from build123d import *

# Parameters (mm, degrees)
SKETCH1_W               = 80
SKETCH1_H               = 90
BOSS_EXTRUDE1_DEPTH     = 6
SKETCH4_W               = 80
SKETCH4_H               = 90
SKETCH4_W_2             = 73
SKETCH4_H_2             = 83
BOSS_EXTRUDE2_DEPTH     = 54
SKETCH6_R               = 4.05
SKETCH6_R_2             = 5
CUT_EXTRUDE1_DEPTH      = 40
SKETCH7_R               = 7
CUT_EXTRUDE2_DEPTH      = 2.8
BOSS_EXTRUDE3_DEPTH     = 7
SKETCH11_R              = 2.85
BOSS_EXTRUDE4_DEPTH     = 2
CUT_EXTRUDE3_DEPTH      = 9
CUT_EXTRUDE3_DEPTH_BACK = 6
SKETCH5_R               = 1.5
CUT_EXTRUDE4_DEPTH      = 6
CUT_EXTRUDE4_DEPTH_BACK = 81.876448982
SKETCH12_W              = 33
SKETCH12_H              = 13.5
CUT_EXTRUDE6_DEPTH      = 3.5
SKETCH17_R              = 8
CUT_EXTRUDE8_DEPTH      = 2
CUT_EXTRUDE9_DEPTH      = 1.5
CUT_EXTRUDE10_DEPTH     = 10
BOSS_EXTRUDE5_DEPTH     = 90
BOSS_EXTRUDE5_2_DEPTH   = 90
SKETCH21_W              = 3.5
SKETCH21_H              = 8
BOSS_EXTRUDE6_DEPTH     = 80
SKETCH22_W              = 80
SKETCH22_H              = 3.5
BOSS_EXTRUDE7_DEPTH     = 4.5
SKETCH24_W              = 8
SKETCH24_H              = 3.5
BOSS_EXTRUDE8_DEPTH     = 90


with BuildPart() as part:
    # Sketch1 → Boss-Extrude1 (new body)
    with BuildSketch(Plane(origin=(0, 0, 0), x_dir=(1, 0, 0), z_dir=(0, 1, 0))):
        Rectangle(SKETCH1_W, SKETCH1_H)
    extrude(amount=BOSS_EXTRUDE1_DEPTH)

    # Sketch4 → Boss-Extrude2 (add)
    with BuildSketch(Plane(origin=(0, 6, 0), x_dir=(1, 0, 0), z_dir=(0, 1, 0))):
        Rectangle(SKETCH4_W, SKETCH4_H)
        Rectangle(SKETCH4_W_2, SKETCH4_H_2, mode=Mode.SUBTRACT)
    extrude(amount=BOSS_EXTRUDE2_DEPTH)

    # Sketch6 → Cut-Extrude1 (cut)
    with BuildSketch(Plane(origin=(0, 6, 0), x_dir=(1, 0, 0), z_dir=(0, 1, 0))):
        with Locations(Location((-20, 25, 0), (0, 0, 270))):
            Circle(SKETCH6_R)
        with Locations(Location((-20, -25, 0), (0, 0, 270))):
            Circle(SKETCH6_R)
        with Locations(Location((20, -25, 0), (0, 0, 270))):
            Circle(SKETCH6_R_2)
    extrude(amount=-CUT_EXTRUDE1_DEPTH, mode=Mode.SUBTRACT)

    # Sketch7 → Cut-Extrude2 (cut)
    with BuildSketch(Plane(origin=(0, 6, 0), x_dir=(1, 0, 0), z_dir=(0, 1, 0))):
        with Locations(Location((-20, 25, 0), (0, 0, 270))):
            Circle(SKETCH7_R)
        with Locations(Location((-20, -25, 0), (0, 0, 270))):
            Circle(SKETCH7_R)
    extrude(amount=-CUT_EXTRUDE2_DEPTH, mode=Mode.SUBTRACT)

    # Sketch10 → Boss-Extrude3 (add)
    with BuildSketch(Plane(origin=(0, 6, 0), x_dir=(1, 0, 0), z_dir=(0, 1, 0))):
        Polygon((-32.5, 29.600297611), (-37.35, 26.800148806), (-37.35, 21.199851194), (-32.5, 18.399702389), (-27.65, 21.199851194), (-27.65, 26.800148806), align=None)
        Polygon((2.8, 19.600297611), (-2.05, 16.800148806), (-2.05, 11.199851194), (2.8, 8.399702389), (7.65, 11.199851194), (7.65, 16.800148806), align=None)
        Polygon((2.8, -8.399702389), (-2.05, -11.199851194), (-2.05, -16.800148806), (2.8, -19.600297611), (7.65, -16.800148806), (7.65, -11.199851194), align=None)
        Polygon((-27.65, -21.199851194), (-32.5, -18.399702389), (-37.35, -21.199851194), (-37.35, -26.800148806), (-32.5, -29.600297611), (-27.65, -26.800148806), align=None)
    extrude(amount=BOSS_EXTRUDE3_DEPTH)

    # Sketch11 → Boss-Extrude4 (add)
    with BuildSketch(Plane(origin=(0, 13, 0), x_dir=(1, 0, 0), z_dir=(0, 1, 0))):
        with Locations(Location((-32.5, 24, 0), (0, 0, 270))):
            Circle(SKETCH11_R)
        with Locations(Location((2.8, 14, 0), (0, 0, 270))):
            Circle(SKETCH11_R)
        with Locations(Location((2.8, -14, 0), (0, 0, 270))):
            Circle(SKETCH11_R)
        with Locations(Location((-32.5, -24, 0), (0, 0, 270))):
            Circle(SKETCH11_R)
    extrude(amount=BOSS_EXTRUDE4_DEPTH)

    # Sketch5 → Cut-Extrude3 (cut, two sides: drawn at the far end of the back side and taken through both)
    with BuildSketch(Plane(origin=(0, 6, 0), x_dir=(1, 0, 0), z_dir=(0, 1, 0)).offset(-CUT_EXTRUDE3_DEPTH_BACK)):
        with Locations(Location((-32.5, 24, 0), (0, 0, 270))):
            Circle(SKETCH5_R)
        with Locations(Location((-32.5, -24, 0), (0, 0, 270))):
            Circle(SKETCH5_R)
        with Locations(Location((2.8, 14, 0), (0, 0, 270))):
            Circle(SKETCH5_R)
        with Locations(Location((2.8, -14, 0), (0, 0, 270))):
            Circle(SKETCH5_R)
    extrude(amount=CUT_EXTRUDE3_DEPTH + CUT_EXTRUDE3_DEPTH_BACK, mode=Mode.SUBTRACT)

    # Sketch8 → Cut-Extrude4 (cut, two sides: drawn at the far end of the back side and taken through both)
    with BuildSketch(Plane(origin=(0, 6, 0), x_dir=(1, 0, 0), z_dir=(0, 1, 0)).offset(-CUT_EXTRUDE4_DEPTH_BACK)):
        Polygon((-29.65, 25.645448267), (-32.5, 27.290896534), (-35.35, 25.645448267), (-35.35, 22.354551733), (-32.5, 20.709103466), (-29.65, 22.354551733), align=None)
        Polygon((-29.65, -22.354551733), (-32.5, -20.709103466), (-35.35, -22.354551733), (-35.35, -25.645448267), (-32.5, -27.290896534), (-29.65, -25.645448267), align=None)
        Polygon((5.65, -12.354551733), (2.8, -10.709103466), (-0.05, -12.354551733), (-0.05, -15.645448267), (2.8, -17.290896534), (5.65, -15.645448267), align=None)
        Polygon((5.65, 15.645448267), (2.8, 17.290896534), (-0.05, 15.645448267), (-0.05, 12.354551733), (2.8, 10.709103466), (5.65, 12.354551733), align=None)
    extrude(amount=CUT_EXTRUDE4_DEPTH + CUT_EXTRUDE4_DEPTH_BACK, mode=Mode.SUBTRACT)

    # Sketch12 → Cut-Extrude6 (cut)
    with BuildSketch(Plane(origin=(-36.5, 0, 0), x_dir=(0, 0, -1), z_dir=(1, 0, 0))):
        with Locations((0, 23.25)):
            Rectangle(SKETCH12_W, SKETCH12_H)
    extrude(amount=-CUT_EXTRUDE6_DEPTH, mode=Mode.SUBTRACT)

    # Sketch17 → Cut-Extrude8 (cut)
    with BuildSketch(Plane.ZY.offset(40)):
        with Locations((0, 45.25)):
            Circle(SKETCH17_R)
    extrude(amount=-CUT_EXTRUDE8_DEPTH, mode=Mode.SUBTRACT)

    # Sketch15 → Cut-Extrude9 (cut)
    with BuildSketch(Plane(origin=(-36.5, 0, 0), x_dir=(0, 0, -1), z_dir=(1, 0, 0))):
        Polygon((-6.495190528, 56.5), (-12.990381057, 45.25), (-6.495190528, 34), (6.495190528, 34), (12.990381057, 45.25), (6.495190528, 56.5), align=None)
    extrude(amount=-CUT_EXTRUDE9_DEPTH, mode=Mode.SUBTRACT)

    # Sketch19 → Cut-Extrude10 (cut)
    with BuildSketch(Plane(origin=(0, 6, 0), x_dir=(1, 0, 0), z_dir=(0, 1, 0))):
        with BuildLine():
            Line((-3.5, -5.5), (-3.5, 5.5))
            ThreePointArc((-3.5, 5.5), (0, 9), (3.5, 5.5))
            Line((3.5, 5.5), (3.5, -5.5))
            ThreePointArc((3.5, -5.5), (0, -9), (-3.5, -5.5))
        make_face()
    extrude(amount=-CUT_EXTRUDE10_DEPTH, mode=Mode.SUBTRACT)



with BuildPart() as body_2:
    # Sketch20 → Boss-Extrude5 (new body)
    with BuildSketch(Plane(origin=(0, 0, -45), x_dir=(-1, 0, 0), z_dir=(0, 0, -1))):
        Polygon((-40, 60), (-36.5, 60), (-36.5, 64.5), (-32, 64.5), (-32, 68), (-40, 68), align=None)
    extrude(amount=-BOSS_EXTRUDE5_DEPTH)


with BuildPart() as body_3:
    # Sketch20 → Boss-Extrude5 2 (new body)
    with BuildSketch(Plane(origin=(0, 0, -45), x_dir=(-1, 0, 0), z_dir=(0, 0, -1))):
        Polygon((40, 60), (36.5, 60), (36.5, 64.5), (32, 64.5), (32, 68), (40, 68), align=None)
    extrude(amount=-BOSS_EXTRUDE5_2_DEPTH)


with BuildPart() as part_1:
    add(part.part)

    add(body_2.part)  # Boss-Extrude6 merges body 2
    # Sketch21 → Boss-Extrude6 (add)
    with BuildSketch(Plane(origin=(40, 0, 0), x_dir=(0, 0, -1), z_dir=(1, 0, 0))):
        with Locations((-43.25, 64)):
            Rectangle(SKETCH21_W, SKETCH21_H)
    extrude(amount=-BOSS_EXTRUDE6_DEPTH)


    add(body_3.part)  # Boss-Extrude7 merges body 3
    # Sketch22 → Boss-Extrude7 (add)
    with BuildSketch(Plane(origin=(0, 0, 41.5), x_dir=(-1, 0, 0), z_dir=(0, 0, -1))):
        with Locations((0, 66.25)):
            Rectangle(SKETCH22_W, SKETCH22_H)
    extrude(amount=BOSS_EXTRUDE7_DEPTH)

    # Sketch24 → Boss-Extrude8 (add)
    with BuildSketch(Plane.XY.offset(45)):
        with Locations((-36, 58.25)):
            Rectangle(SKETCH24_W, SKETCH24_H)
        with Locations((36, 58.25)):
            Rectangle(SKETCH24_W, SKETCH24_H)
    extrude(amount=-BOSS_EXTRUDE8_DEPTH)


solid = part_1.part
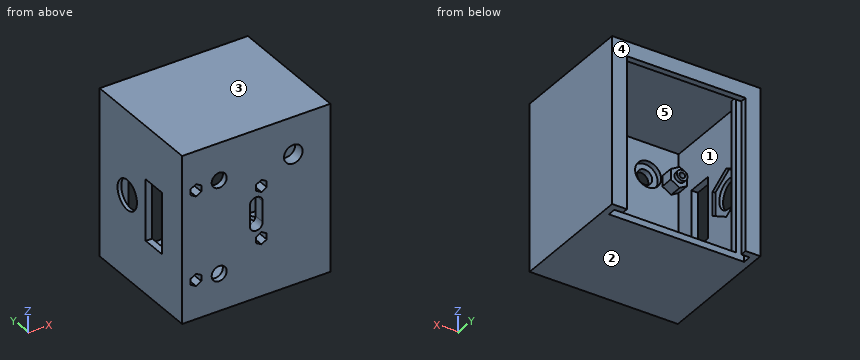
Part model, mm, in its own coordinate system. Face numbers are marked on the shaded views. A direction names the side the tool comes from. Coordinates: 2 decimals unless noted, no trailing zeros. Loops run counter-clockwise (first coordinate to the right, second up) from the corner with the lowest first, then second, coordinate; pieces in that order, holes last. Notation, with made-up numbers: M 71,27.25 L 99,27.25 A7 ccw 99,39.25 Z; hole C 63.25,85 d6. An arc over 180 degrees is marked long. Use a Markdown table: item, result. Add a question column.
Q1. Cut at C-C (x = 30). Write the cut outline in (y, z).
Q2. Mould opens along Y. For the marked faces 3, 4 and 5 say: +Y half, -Y half, draft (parallel to the pull), parting line (faces both ways), or undercut.
Q3. Pin check, flat tips, straight feed: P1, Ø6.5, axis at x = 3.5, z = -15.5, coming from the +Y side; P2, Ø1.5, axis at y = 22.5, z = 4.5, coming from the -X side; P3, Ø4, axis at x = -32.5, z = -24, coming from the -Y side. Stop position of each tip, or through.
Q4. Which spindle directions (+Z, -Z, +X, -X, +Y, -Y) get a long thin tool onto all of the face, cutting with end or side? Do the marked faces 1 and 2. Say none if no direction does.
Q5. Probe L1, parallel to X at y = 13.25, z = -24; L2, parallel to X at y = 12.95, z = -14; L3, parallel to Y at x = 35, z = 2. List the from-to ranges inside material, lowest first.
Q6. Cut at D-D (z = -36.5). Write the cut outline in (x, y).
Q7. Cut at A-A (z = 0). Give the number of separate pieces and of enclosed holes in the cut face, and give its area (3 significant figures).
Q8. Cut at B-B (y = 58.5). Write the cut outline in (x, z), and give its area (3 significant figures).
Worked out:
| question | item | result |
|---|---|---|
| 1 | outline | M 0,-45 L 60,-45 L 60,-41.5 L 6,-41.5 L 6,41.5 L 64.5,41.5 L 64.5,37 L 68,37 L 68,45 L 0,45 Z |
| 2 | face 3 | draft |
| 2 | face 4 | +Y half |
| 2 | face 5 | undercut |
| 3 | P1 | stops at y = 15 |
| 3 | P2 | stops at x = 36.5 |
| 3 | P3 | stops at y = 12 |
| 4 | face 1 | none |
| 4 | face 2 | -Z, +X, -X, +Y, -Y |
| 5 | L1 | x = -40 to -36.5, -35.35 to -34, -31 to -29.65, 36.5 to 40 |
| 5 | L2 | x = -40 to -36.5, -2.05 to 1.3, 4.3 to 7.65, 36.5 to 40 |
| 5 | L3 | y = 0 to 6, 56.5 to 60, 64.5 to 68 |
| 6 | outline | M -40,0 L 40,0 L 40,68 L 32,68 L 32,64.5 L 36.5,64.5 L 36.5,60 L 32,60 L 32,56.5 L 36.5,56.5 L 36.5,6 L -36.5,6 L -36.5,56.5 L -32,56.5 L -32,60 L -36.5,60 L -36.5,64.5 L -32,64.5 L -32,68 L -40,68 Z |
| 7 | separate pieces | 4 |
| 7 | enclosed holes | 0 |
| 7 | area | 822 mm2 |
| 8 | outline | M -40,-45 L 40,-45 L 40,45 L -40,45 Z; hole M -32,-41.5 L 32,-41.5 L 32,41.5 L -32,41.5 Z |
| 8 | area | 1,890 mm2 |
